from build123d import *

# Parameters (mm, degrees)
SKETCH1_W           = 393.7
SKETCH1_H           = 393.7
BOSS_EXTRUDE1_DEPTH = 19.05
CUT_EXTRUDE2_DEPTH  = 1
SKETCH3_R           = 4.365625
CUT_EXTRUDE4_DEPTH  = 12.5
FILLET1_R           = 2


with BuildPart() as part:
    # Sketch1 → Boss-Extrude1 (new body)
    with BuildSketch(Plane.XY):
        with Locations((196.85, 196.85)):
            Rectangle(SKETCH1_W, SKETCH1_H)
    extrude(amount=BOSS_EXTRUDE1_DEPTH)

    # Sketch2 → Cut-Extrude2 (cut)
    with BuildSketch(Plane.XY.offset(19.05)):
        with BuildLine():
            Line((55.8, 50.8), (198.2, 50.8))
            ThreePointArc((198.2, 50.8), (206.735533906, 47.264466094), (203.2, 55.8))
            Line((203.2, 55.8), (203.2, 122.254))
            ThreePointArc((203.2, 122.254), (206.735533906, 130.789533906), (198.2, 127.254))
            Line((198.2, 127.254), (55.8, 127.254))
            ThreePointArc((55.8, 127.254), (47.264466094, 130.789533906), (50.8, 122.254))
            Line((50.8, 122.254), (50.8, 55.8))
            ThreePointArc((50.8, 55.8), (47.264466094, 47.264466094), (55.8, 50.8))
        make_face()
    extrude(amount=-CUT_EXTRUDE2_DEPTH, mode=Mode.SUBTRACT)

    # Sketch3 → Cut-Extrude4 (cut)
    with BuildSketch(Plane.XY.offset(18.05)):
        with Locations((61.2, 89.2)):
            Circle(SKETCH3_R)
        with Locations((91.4, 89.2)):
            Circle(SKETCH3_R)
        with Locations((76.2, 75)):
            Circle(SKETCH3_R)
        with Locations((76.2, 103.2)):
            Circle(SKETCH3_R)
    extrude(amount=-CUT_EXTRUDE4_DEPTH, mode=Mode.SUBTRACT)

    # Fillet1
    fillet1_edges = [part.edges().sort_by_distance(p)[0] for p in [
        (203.2, 55.8, 18.55),
        (198.2, 50.8, 18.55),
        (55.8, 50.8, 18.55),
        (50.8, 55.8, 18.55),
        (50.8, 122.254, 18.55),
        (55.8, 127.254, 18.55),
        (198.2, 127.254, 18.55),
        (203.2, 122.254, 18.55),
    ]]
    fillet(fillet1_edges, radius=FILLET1_R)


solid = part.part
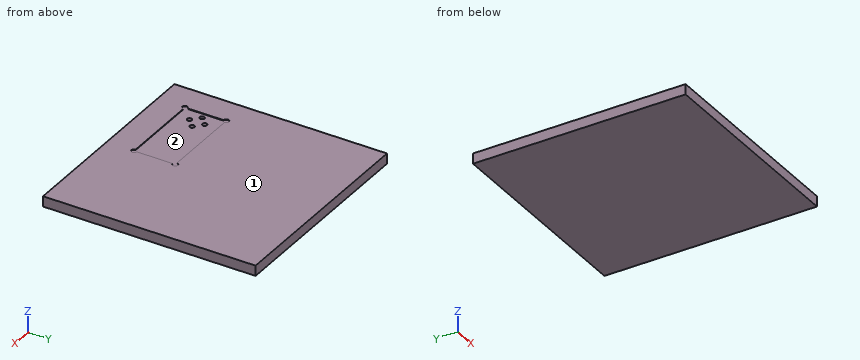
Verification items for the finished model (mm, model axes). Face numbers are marked on the shaded views. Give positions to 0.01 mm unless a question says otherwise; leave off trailing zeros.
(1) Material ranges on line 1 (Y direction, x = 91.4, z = 14.5); line 2 (Y direction, x = 60.5, z = 15); line 3 (Z direction, x = 143, y = 112), recorded low to high.
(2) Mould release check, pull along Y, two halves, no side actions. Record for the marked faces 1 and 2: +Y half, -Y half, draft (parallel to the pull), parting line (faces both ways), or undercut.
(3) Gauge pin test, flat ends, axial feed: pin 1 (4.5 mm diameter, centred on x = 92, y = 89, fed in from +Z); pin 2 (7 mm diameter, centred on x = 78, y = 101, fed in from +Z). Record the tip position at first contact, or that the pin passes through.
Worked out:
1. line 1: y = 0 to 84.83, 93.57 to 393.7
1. line 2: y = 0 to 84.89, 93.51 to 393.7
1. line 3: z = 0 to 18.05
2. face 1: draft
2. face 2: undercut
3. pin 1: stops at z = 5.55
3. pin 2: stops at z = 18.05
